Build history of the part. All positions in model axes, mm. A direction names the side the tool comes from. Coordinates: 2 decimals unless noted, no trailing zeros. Loops run counter-clockwise (first coordinate to the right, second up) from the corner with the lowest first, then second, coordinate; pieces in that order, holes last.
(1) Slice it at A-A (y = -24). Give the cut face in (x, z), and give its area (3 significant figures).
(2) Flat gauge pins, fed straight in: P1, Ø21, axis at x = 60, z = 52, coming from the -Y side; P2, Ø2.5, axis at x = -102, z = 72.5, coming from the -Y side; P3, Ø5, axis at x = -9, y = 51, coming from the +Z side. Where does each tip first touch, or does it go through?
(3) Two-plate mould, pull along Y, no slides. Class faces 4 (the face through (-65.38, 77.15, 64.22)), 5 (the face through (-64, -78.5, 61)), 6 (the face through (-93, 1, 82)): pulls with the +Y half, pulls with the -Y half, needs draft (parallel to the pull), parting line crosses it, or undercut.
(4) Slice it at C-C (z = 75.5). Give the cut face in (x, y), and give its area (3 significant figures).
(5) Wall check: L1, parallel to X at y = -74, z = 52; L2, parallel to Y at x = 4.5, z = 32; L3, parallel to Z at x = -63.88, y = 75.25. Give the ranges that are in metal, low to high.
(6) Tool access for faces 1 (the face through (-103.5, 1, 36)), 2 (the face through (74.503, -73.204, 57.225)), 3 (the face through (71.231, 70.246, 55.135)): list every direction of +Z, -Z, +X, -X, +Y, -Y with a clear straight run to the whole face (end or side of a thin tool).
(7) Slice it at D-D (z = 27). Give the cut face in (x, y).
(8) Slice it at B-B (x = -92.5). Give the cut face in (y, z), and give its area (3 significant figures).
Autodesk Inventor part; units mm, degrees
ref_plane "РабПлоскость2" through (-75.6513, -84.5, 41.0487) normal (0, -1, 0) x (0.941, 0, -0.3385)
ref_plane "РабПлоскость3" through (-75.6513, -78.5, 41.0487) normal (0, 1, 0) x (0.3385, 0, 0.941)
ref_plane "РабПлоскость4" through (51.3812, -70.5, 40.3212) normal (0, 1, 0) x (0.4829, 0, 0.8757)
ref_plane "РабПлоскость1" through (0, 0, 10) normal (0, 0, 1) x (1, 0, 0)
sketch "Эскиз1" plane through (0, 0, 10) normal (0, 0, 1) x (1, 0, 0)
  line L0 (-107.5, 70) -> (107.5, 70)
  line L1 (107.5, 70) -> (107.5, -70)
  line L2 (107.5, -70) -> (-107.5, -70)
  line L3 (-107.5, -70) -> (-107.5, 70)
  line L4 (-107.5, 70) -> (107.5, -70) construction
  line L5 (107.5, 70) -> (-107.5, -70) construction
  point P0 (0, 0)
  dimension "d1" = 215
  dimension "d2" = 140
extrude "Выдавливание1" add sketch "Эскиз1" along normal blind 7
sketch "Эскиз2" plane through (-107.5, 70, 10) normal (0, 1, 0) x (1, 0, 0)
  line L0 (215, 0) -> (0, 0)
  line L1 (0, 0) -> (0, -7)
  line L2 (215, -7) -> (0, -7)
  line L3 (215, 0) -> (215, -7)
  line L4 (154.9795, -76.2499) -> (152.5795, -76.2499)
  line L5 (155.2294, -76) -> (154.9795, -76.2499)
  line L6 (159.8295, -76) -> (155.2294, -76)
  line L7 (160.0795, -76.2499) -> (159.8295, -76)
  line L8 (162.4795, -76.2499) -> (160.0795, -76.2499)
  line L9 (162.7294, -76) -> (162.4795, -76.2499)
  line L10 (167.3295, -76) -> (162.7294, -76)
  line L11 (167.5795, -76.2499) -> (167.3295, -76)
  line L12 (169.9795, -76.2499) -> (167.5795, -76.2499)
  line L13 (170.2294, -76) -> (169.9795, -76.2499)
  line L14 (174.8295, -76) -> (170.2294, -76)
  line L15 (175.0795, -76.2499) -> (174.8295, -76)
  line L16 (177.4795, -76.2499) -> (175.0795, -76.2499)
  line L17 (177.7294, -76) -> (177.4795, -76.2499)
  line L18 (182.3295, -76) -> (177.7294, -76)
  line L19 (182.5795, -76.2499) -> (182.3295, -76)
  line L20 (184.9795, -76.2499) -> (182.5795, -76.2499)
  line L21 (185.2294, -76) -> (184.9795, -76.2499)
  line L22 (189.8295, -76) -> (185.2294, -76)
  line L23 (190.0795, -76.2499) -> (189.8295, -76)
  line L24 (192.4795, -76.2499) -> (190.0795, -76.2499)
  line L25 (192.7294, -76) -> (192.4795, -76.2499)
  line L26 (197.3295, -76) -> (192.7294, -76)
  line L27 (197.5795, -76.2499) -> (197.3295, -76)
  line L28 (199.9795, -76.2499) -> (197.5795, -76.2499)
  line L29 (200.2294, -76) -> (199.9795, -76.2499)
  line L30 (204.8295, -76) -> (200.2294, -76)
  line L31 (205.0795, -76.2499) -> (204.8295, -76)
  line L32 (207.4152, -76.2499) -> (205.0795, -76.2499)
  arc A0 (208.0813, -72.8208) -> (207.4152, -76.2499) centre (232.2295, -79.2913) ccw
  line L33 (208.0813, -72.8208) -> (215, -47)
  line L34 (215, -22) -> (215, -47)
  line L35 (215, -22) -> (211, -22)
  line L36 (211, -22) -> (211, -46.4734)
  line L37 (211, -46.4734) -> (204.1602, -72)
  line L38 (204.1602, -72) -> (150.3397, -72)
  line L39 (150.3397, -72) -> (150.3397, -76)
  line L40 (152.3295, -76) -> (150.3397, -76)
  line L41 (152.5795, -76.2499) -> (152.3295, -76)
  line L42 (107.5, 0) -> (107.5, -94.8503)
  line L43 (15.0205, -76.2499) -> (17.4205, -76.2499)
  line L44 (7.5848, -76.2499) -> (9.9205, -76.2499)
  arc A1 (7.5848, -76.2499) -> (6.9187, -72.8208) centre (-17.2295, -79.2913) ccw
  line L45 (6.9187, -72.8208) -> (0, -47)
  line L46 (0, -22) -> (0, -47)
  line L47 (0, -22) -> (4, -22)
  line L48 (4, -22) -> (4, -46.4734)
  line L49 (4, -46.4734) -> (10.8398, -72)
  line L50 (10.8398, -72) -> (64.6603, -72)
  line L51 (215, -22) -> (211, -22)
  line L52 (211, -22) -> (211, -7)
  line L53 (211, -7) -> (215, -7)
  line L54 (215, -7) -> (215, -22)
  line L55 (4, -22) -> (0, -22)
  line L56 (0, -22) -> (0, -7)
  line L57 (0, -7) -> (4, -7)
  line L58 (4, -7) -> (4, -22)
  line L59 (17.8835, -76.2499) -> (7.5848, -76.2499)
  line L60 (10.8398, -72) -> (17.8835, -72)
  line L61 (17.8835, -72) -> (17.8835, -76.2499)
  point P0 (107.5, 10)
  point P1 (17.8835, -72)
extrude "Выдавливание2" add sketch "Эскиз2" against normal up to surface (140 mm away) contours L54 L35 L52 L2 | L2 L58 L47 L56 | L47 L48 L49 L50 L61 L59 L43 L44 A1 L45 L46
sketch "Эскиз3" plane through (-107.5, -70, 10) normal (0, -1, 0) x (1, 0, 0)
  line L0 (0, 0) -> (215, 0)
  line L1 (215, 0) -> (215, 22)
  line L2 (211, 22) -> (215, 22)
  line L3 (211, 7) -> (211, 22)
  line L4 (4, 7) -> (211, 7)
  line L5 (4, 46.4734) -> (4, 7)
  line L6 (10.8398, 72) -> (4, 46.4734)
  line L7 (17.8835, 72) -> (10.8398, 72)
  line L8 (17.8835, 76.2499) -> (17.8835, 72)
  line L9 (7.5848, 76.2499) -> (17.8835, 76.2499)
  arc A0 (6.9187, 72.8208) -> (7.5848, 76.2499) centre (-17.2295, 79.2913) ccw
  line L10 (0, 47) -> (6.9187, 72.8208)
  line L11 (0, 0) -> (0, 47)
  line L12 (205.0795, 76.2499) -> (207.4152, 76.2499)
  line L13 (204.8295, 76) -> (205.0795, 76.2499)
  line L14 (200.2294, 76) -> (204.8295, 76)
  line L15 (199.9795, 76.2499) -> (200.2294, 76)
  line L16 (197.5795, 76.2499) -> (199.9795, 76.2499)
  line L17 (197.3295, 76) -> (197.5795, 76.2499)
  line L18 (192.7294, 76) -> (197.3295, 76)
  line L19 (192.4795, 76.2499) -> (192.7294, 76)
  line L20 (190.0795, 76.2499) -> (192.4795, 76.2499)
  line L21 (189.8295, 76) -> (190.0795, 76.2499)
  line L22 (185.2294, 76) -> (189.8295, 76)
  line L23 (184.9795, 76.2499) -> (185.2294, 76)
  line L24 (182.5795, 76.2499) -> (184.9795, 76.2499)
  line L25 (182.3295, 76) -> (182.5795, 76.2499)
  line L26 (177.7294, 76) -> (182.3295, 76)
  line L27 (177.4795, 76.2499) -> (177.7294, 76)
  line L28 (175.0795, 76.2499) -> (177.4795, 76.2499)
  line L29 (174.8295, 76) -> (175.0795, 76.2499)
  line L30 (170.2294, 76) -> (174.8295, 76)
  line L31 (169.9795, 76.2499) -> (170.2294, 76)
  line L32 (167.5795, 76.2499) -> (169.9795, 76.2499)
  line L33 (167.3295, 76) -> (167.5795, 76.2499)
  line L34 (162.7294, 76) -> (167.3295, 76)
  line L35 (162.4795, 76.2499) -> (162.7294, 76)
  line L36 (160.0795, 76.2499) -> (162.4795, 76.2499)
  line L37 (159.8295, 76) -> (160.0795, 76.2499)
  line L38 (155.2294, 76) -> (159.8295, 76)
  line L39 (154.9795, 76.2499) -> (155.2294, 76)
  line L40 (152.5795, 76.2499) -> (154.9795, 76.2499)
  line L41 (152.3295, 76) -> (152.5795, 76.2499)
  line L42 (150.3397, 76) -> (152.3295, 76)
  line L43 (150.3397, 72) -> (150.3397, 76)
  line L44 (150.3397, 72) -> (204.1602, 72)
  line L45 (204.1602, 72) -> (211, 46.4734)
  line L46 (211, 46.4734) -> (211, 22)
  line L47 (211, 22) -> (215, 22)
  line L48 (215, 22) -> (215, 47)
  line L49 (215, 47) -> (208.0813, 72.8208)
  arc A1 (207.4152, 76.2499) -> (208.0813, 72.8208) centre (232.2295, 79.2913) ccw
  line L50 (17.8835, 76.2499) -> (207.9879, 76)
  line L51 (17.8835, 72) -> (150.3397, 72)
  circle A2 centre (43.62, 42.82) radius 4
  circle A3 centre (171.38, 42.82) radius 4.3
  point P0 (107.5, -10)
extrude "Выдавливание3" add sketch "Эскиз3" against normal blind 6 contours L3 L4 L5 L6 L7 L51 L44 L45 L46
sketch "Эскиз4" plane through (-107.5, -70, 10) normal (0, -1, 0) x (1, 0, 0)
  circle A0 centre (43.62, 42.82) radius 9.5
  circle A1 centre (43.62, 42.82) radius 11.5
  point P0 (107.5, -10)
  dimension "d9" = 23
ref_plane "РабПлоскость2" through (-75.6513, -84.5, 41.0487) normal (0, -1, 0) x (0.941, 0, -0.3385)
extrude "Выдавливание4" add sketch "Эскиз4" along normal up to surface (14.5 mm away)
sketch "Эскиз5" plane through (-63.88, -70, 52.82) normal (0, -1, 0) x (1, 0, 0)
  circle A0 centre (0, 0) radius 7.707
  circle A1 centre (0, 0) radius 9.5
  point P0 (63.88, -52.82)
ref_plane "РабПлоскость3" through (-75.6513, -78.5, 41.0487) normal (0, 1, 0) x (0.3385, 0, 0.941)
extrude "Выдавливание5" add sketch "Эскиз5" along normal up to surface (8.5 mm away)
sketch "Эскиз6" plane through (-107.5, -70, 10) normal (0, -1, 0) x (1, 0, 0)
  point P0 (107.5, -10)
sketch "Эскиз7" plane through (-107.5, -70, 10) normal (0, -1, 0) x (1, 0, 0)
  circle A0 centre (171.38, 42.82) radius 7.707
  circle A1 centre (171.38, 42.82) radius 9.5
  point P0 (107.5, -10)
ref_plane "РабПлоскость4" through (51.3812, -70.5, 40.3212) normal (0, 1, 0) x (0.4829, 0, 0.8757)
extrude "Выдавливание6" add sketch "Эскиз7" along normal up to surface (0.5 mm away)
sketch "Эскиз8" plane through (-107.5, -70, 10) normal (0, -1, 0) x (1, 0, 0)
  circle A0 centre (171.38, 42.82) radius 9.5
  circle A1 centre (171.38, 42.82) radius 11.5
  point P0 (107.5, -10)
  dimension "d16" = 23
ref_plane "РабПлоскость5" through (51.3812, -76.5, 40.3212) normal (0, -1, 0) x (0.8757, 0, -0.4829)
extrude "Выдавливание7" add sketch "Эскиз8" along normal up to surface (6.5 mm away)
mirror "Зеркальное отражение1" about plane through (0, 0, 0) normal (0, 1, 0) of "Выдавливание3", "Выдавливание4", "Выдавливание5", "Выдавливание6", "Выдавливание7"
sketch "Эскиз9" plane through (-107.5, -70, 10) normal (-1, 0, 0) x (0, 0, 1)
  line L0 (69.9727, 77.7173) -> (54.1331, 77.7173)
  line L1 (54.1331, 77.7173) -> (54.1331, 23.438)
  line L2 (54.1331, 23.438) -> (69.9727, 23.438)
  line L3 (69.9727, 23.438) -> (69.9727, 77.7173)
  point P0 (-10, 70)
extrude "Выдавливание8" cut sketch "Эскиз9" against normal blind 10
ref_plane "РабПлоскость6" through (-75.6513, 84.5, 41.0487) normal (0, -1, 0) x (0.941, 0, -0.3385)
ref_plane "РабПлоскость7" through (-75.6513, 78.5, 41.0487) normal (0, 1, 0) x (0.3385, 0, 0.941)
ref_plane "РабПлоскость8" through (51.3812, 70.5, 40.3212) normal (0, 1, 0) x (0.4829, 0, 0.8757)
ref_plane "РабПлоскость9" through (51.3812, 76.5, 40.3212) normal (0, -1, 0) x (0.8757, 0, -0.4829)
Response values:
1. outline: (-107.5, 10) - (107.5, 10) - (107.5, 32) - (103.5, 32) - (103.5, 17) - (-103.5, 17) - (-103.5, 56.47) - (-101.45, 64.13) - (-105.59, 64.13) - (-107.5, 57) - close; (-101.34, 79.97) - (-97.5, 79.97) - (-97.5, 78.87) - (-96.66, 82) - (-89.62, 82) - (-89.62, 86.25) - (-99.92, 86.25) arc R25.01 cw to (-100.58, 82.82) - close
1. area: 1,810 mm2
2. P1: stops at y = -76.5
2. P2: stops at y = -70
2. P3: stops at z = 17
3. face 4: needs draft
3. face 5: pulls with the -Y half
3. face 6: undercut
4. outline: (-102.54, -70) - (98.4, -70) - (98.4, -64) - (-98.4, -64) - (-98.4, -46.56) - (-102.54, -46.56) - close; (-102.54, 7.72) - (-98.4, 7.72) - (-98.4, 64) - (98.4, 64) - (98.4, 70) - (-102.54, 70) - close
4. area: 2,720 mm2
5. L1: x = -75.35 to -71.54, -56.22 to -52.41, 52.41 to 54.42, 73.34 to 75.35
5. L2: y = -70 to -64, 64 to 70
5. L3: z = 41.32 to 45.11, 60.53 to 64.32
6. face 1: none
6. face 2: -Y
6. face 3: +Y
7. outline: (-107.5, -70) - (107.5, -70) - (107.5, 70) - (-107.5, 70) - close; hole (-103.5, -64) - (103.5, -64) - (103.5, 64) - (-103.5, 64) - close
8. outline: (-70, 10) - (70, 10) - (70, 86.25) - (-70, 86.25) - close; hole (-64, 17) - (64, 17) - (64, 82) - (-64, 82) - close
8. area: 2,350 mm2
